from build123d import *

# Parameters (mm, degrees)
F1_DEPTH = 75
F2_R     = 5
F3_R     = 25.635066
F4_DEPTH = 25


with BuildPart() as f1:
    # F0 (on Front) → F1 (new body)
    with BuildSketch(Plane.XZ):
        with BuildLine():
            Line((24.407001, 77.690751), (-25.592999, 77.690751))
            ThreePointArc((-25.592999, 77.690751), (-43.270669, 70.36842), (-50.592999, 52.690751))
            Line((-50.592999, 52.690751), (-50.592999, 2.690751))
            ThreePointArc((-50.592999, 2.690751), (-43.270669, -14.986919), (-25.592999, -22.309249))
            Line((-25.592999, -22.309249), (24.407001, -22.309249))
            ThreePointArc((24.407001, -22.309249), (42.08467, -14.986919), (49.407001, 2.690751))
            Line((49.407001, 2.690751), (49.407001, 52.690751))
            ThreePointArc((49.407001, 52.690751), (42.08467, 70.36842), (24.407001, 77.690751))
        make_face()
    extrude(amount=F1_DEPTH)

    # F2
    f2_edges = [f1.edges().sort_by_distance(p)[0] for p in [
        (24.407001, -37.5, 77.690751),
        (-0.592999, -75, 77.690751),
        (42.08467, -75, 70.36842),
        (-50.592999, -37.5, 2.690751),
        (-50.592999, 0, 27.690751),
        (-43.270669, 0, -14.986919),
        (42.08467, 0, 70.36842),
        (49.407001, 0, 27.690751),
        (-0.592999, 0, 77.690751),
        (-43.270669, 0, 70.36842),
        (-0.592999, 0, -22.309249),
        (42.08467, 0, -14.986919),
    ]]
    fillet(f2_edges, radius=F2_R)

    # F3 (on face) → F4 (cut)
    with BuildSketch(Plane.XZ.offset(75)):
        with Locations((-3.018171, 28.991828)):
            Circle(F3_R)
    extrude(amount=-F4_DEPTH, mode=Mode.SUBTRACT)


solid = f1.part
Model file for the job. Use its own axes, mm. A direction names the side the tool comes from. Give positions to 0.01 mm unless a question says otherwise; leave off trailing zeros. Loops run counter-clockwise (first coordinate to the right, second up) from the corner with the lowest first, then second, coordinate; pieces in that order, holes last.
1) Saw through at D-D (x = -9). Write the cut outline in (y, z), plus the area to 3 significant figures.
2) Saw through at B-B (x = 4.5). Write the cut outline in (y, z), plus the area to 3 significant figures.
3) Flat gauge pins, fed straight in: pin 1 Ø15.5 at (x, z) = (-0.5, 23.5) entering from -Y; pin 2 Ø5 at (y, z) = (-40.5, 67) entering from -X. Where does each tip first touch, or does it go through?
4) Saw through at C-C (y = -43). Write the cut outline in (x, z), plus the area to 3 significant figures.
5) Wall check: line 1 (Y direction, x = -11, z = 49.5); line 2 (Z direction, x = -21.5, y = -56); line 3 (Z direction, x = -10, y = -4.5). Give the ranges that are in metal, low to high.
6) Tool access for faces 4 (the flat face through (-3, -50, 29)), 5 (the cylindrical face through (-43.464, -37.045, -14.791)): list every direction of +Z, -Z, +X, -X, +Y, -Y with a clear straight run to the whole face (end or side of a thin tool).
7) Saw through at A-A (y = -66). Write the cut outline in (x, z).
8) Pull direction X, two halves, no side cores. Call faces 1 (the flat face through (-1, 0, 28)), 2 (the cylindrical face through (-21.91, -62.68, 46.32)), 3 (the cylindrical face through (-49.167, -1.504, 27.341)): +X half, -X half, draft (parallel to the pull), parting line (faces both ways), or undercut.
Answer block:
1. outline: (-75, -17.31) arc R5 ccw to (-70, -22.31) - (-5, -22.31) arc R5 ccw to (0, -17.31) - (0, 72.69) arc R5 ccw to (-5, 77.69) - (-70, 77.69) arc R5 ccw to (-75, 72.69) - (-75, 53.92) - (-50, 53.92) - (-50, 4.06) - (-75, 4.06) - close
1. area: 6,230 mm2
2. outline: (-75, -17.31) arc R5 ccw to (-70, -22.31) - (-5, -22.31) arc R5 ccw to (0, -17.31) - (0, 72.69) arc R5 ccw to (-5, 77.69) - (-70, 77.69) arc R5 ccw to (-75, 72.69) - (-75, 53.5) - (-50, 53.5) - (-50, 4.48) - (-75, 4.48) - close
2. area: 6,250 mm2
3. pin 1: stops at y = -50
3. pin 2: stops at x = -47.63
4. outline: (-50.59, 2.69) arc R25 ccw to (-25.59, -22.31) - (24.41, -22.31) arc R25 ccw to (49.41, 2.69) - (49.41, 52.69) arc R25 ccw to (24.41, 77.69) - (-25.59, 77.69) arc R25 ccw to (-50.59, 52.69) - close
4. area: 9,460 mm2
5. line 1: y = -50 to 0
5. line 2: z = -22.31 to 11.23, 46.76 to 77.69
5. line 3: z = -22.28 to 77.67
6. face 4: -Y
6. face 5: -Z, -X, +Y, -Y
7. outline: (-50.59, 2.69) arc R25 ccw to (-25.59, -22.31) - (24.41, -22.31) arc R25 ccw to (49.41, 2.69) - (49.41, 52.69) arc R25 ccw to (24.41, 77.69) - (-25.59, 77.69) arc R25 ccw to (-50.59, 52.69) - close; hole circle Ø51.27 at (-3.02, 28.99)
8. face 1: draft
8. face 2: undercut
8. face 3: -X half
